```python
from build123d import *

# Parameters (mm, degrees)
SKETCH1_R           = 2.75
BOSS_EXTRUDE1_DEPTH = 5
CHAMFER1_SIZE       = 3


with BuildPart() as part:
    # Sketch1 → Boss-Extrude1 (new body)
    with BuildSketch(Plane.XY.offset(847.256699138)):
        Polygon((445.331056746, -16.940654003), (425.331056746, -16.940654003), (393.576791941, -71.940654003), (393.576791941, -91.940654003), (445.331056746, -91.940654003), align=None)
        with Locations(Location((435.331056746, -28.311683021, 0), (0, 0, 180))):
            Circle(SKETCH1_R, mode=Mode.SUBTRACT)
        with Locations(Location((435.331056746, -64.663237098, 0), (0, 0, 180))):
            Circle(SKETCH1_R, mode=Mode.SUBTRACT)
        with Locations(Location((400.469639923, -81.940654003, 0), (0, 0, 180))):
            Circle(SKETCH1_R, mode=Mode.SUBTRACT)
        with Locations(Location((435.331056746, -81.940654003, 0), (0, 0, 180))):
            Circle(SKETCH1_R, mode=Mode.SUBTRACT)
    extrude(amount=-BOSS_EXTRUDE1_DEPTH)

    # Chamfer1
    chamfer1_edges = [part.edges().sort_by_distance(p)[0] for p in [
        (445.331056746, -91.940654003, 844.756699138),
        (393.576791941, -91.940654003, 844.756699138),
        (425.331056746, -16.940654003, 844.756699138),
        (445.331056746, -16.940654003, 844.756699138),
    ]]
    chamfer(chamfer1_edges, length=CHAMFER1_SIZE)


solid = part.part
```
For this review, take the finished solid that the model builds, in its own axes (mm). Coordinates: 2 decimals unless noted, no trailing zeros. Loops run counter-clockwise (first coordinate to the right, second up) from the corner with the lowest first, then second, coordinate; pieces in that order, holes last. Notation, with made-up numbers: (88.25, 29.5) -> (124.25, 29.5) arc R18 cw to (124.25, 63.5) -> close; hole circle Ø7 at (27.25, 72.25). An arc over 180 degrees is marked (long way). Return JSON: item names as keys, results as strings. Group by question number.
(1) Consider section A-A, the plane y = -83. Give the boundary of the cut face in (x, z), plus the area to 3 significant figures.
(2) Consider section D-D, the plane y = -63. Give the boundary of the cut face in (x, z).
(3) Consider section C-C, the plane z = 846.3. Give the boundary of the cut face in (x, y), plus the area to 3 significant figures.
(4) To check wall thickness, follow L1, parallel to X at y = -83.5, z = 846; L2, parallel to X at y = -81.5, z = 846.2; L3, parallel to Y at x = 402, z = 842.8. State the ranges of each line that lie inside material, in increasing order.
(5) For pin 1 Ø4.5 at (x, y) = (400.47, -81.94) entering from -Z; pin 2 Ø1 at (x, z) = (399.5, 845) entering from +Y, all flat-tipped, find the tip position at first contact; note any pin that passes through.
(6) Consider section B-B, the plane x = 401.5. Give the boundary of the cut face in (y, z), plus the area to 3 significant figures.
(7) Mouldability with a two-part tool opening along Y and no side actions: class faces 1 (the flat face through (408.9, -45.4, 844.8)), 2 (the cylindrical face through (432.71, -29.14, 844.79)), 3 (the flat face through (419, -91.941, 845)) as pulls with the +Y half, pulls with the -Y half, needs draft (parallel to the pull), parting line crosses it, or undercut.
Results below:
{
 "1": {"outline": "(393.58, 842.26) -> (397.93, 842.26) -> (397.93, 847.26) -> (393.58, 847.26) -> close; (403.01, 842.26) -> (432.79, 842.26) -> (432.79, 847.26) -> (403.01, 847.26) -> close; (437.87, 842.26) -> (445.33, 842.26) -> (445.33, 847.26) -> (437.87, 847.26) -> close", "area": "208 mm2"},
 "2": {"outline": "(398.74, 842.26) -> (433.14, 842.26) -> (433.14, 847.26) -> (398.74, 847.26) -> close; (437.52, 842.26) -> (445.33, 842.26) -> (445.33, 847.26) -> (437.52, 847.26) -> close"},
 "3": {"outline": "(393.58, -88.94) -> (396.58, -91.94) -> (442.33, -91.94) -> (445.33, -88.94) -> (445.33, -19.94) -> (442.33, -16.94) -> (428.33, -16.94) -> (423.83, -19.54) -> (393.58, -71.94) -> close; hole circle Ø5.5 at (400.47, -81.94); hole circle Ø5.5 at (435.33, -81.94); hole circle Ø5.5 at (435.33, -64.66); hole circle Ø5.5 at (435.33, -28.31)", "area": "2,900 mm2"},
 "4": {"L1": "x = 393.58 to 398.2, 402.73 to 433.07, 437.6 to 445.33", "L2": "x = 393.58 to 397.76, 403.18 to 432.62, 438.05 to 445.33", "L3": "y = -91.94 to -84.23, -79.66 to -57.35"},
 "5": {"pin 1": "passes through", "pin 2": "stops at y = -60.82"},
 "6": {"outline": "(-91.94, 842.26) -> (-84.49, 842.26) -> (-84.49, 847.26) -> (-91.94, 847.26) -> close; (-79.39, 842.26) -> (-58.22, 842.26) -> (-58.22, 847.26) -> (-79.39, 847.26) -> close", "area": "143 mm2"},
 "7": {"face 1": "pulls with the +Y half", "face 2": "undercut", "face 3": "pulls with the -Y half"}
}
